```python
from build123d import *

# Parameters (mm, degrees)
BASE_FLANGE1_DEPTH          = 3.2639
F_1_4_START                 = -3.2639
F_1_4_CLEARANCE_SLOT1_DEPTH = 3.2639
SKETCH9_W                   = 1.5875
SKETCH9_H                   = 50.8
CUT_EXTRUDE1_DEPTH          = 274.80079868
FILLET1_R                   = 6.35
FILLET2_R                   = 19.05
FILLET3_R                   = 6.35
FILLET4_R                   = 1.5875
F_1_4_CLEARANCE_SLOT2_DEPTH = 3.2639
F_1_4_CLEARANCE_SLOT3_DEPTH = 3.2639


# Read off the part's stored shape, not the designer's step: 1/4 Clearance Slot1, 1/4 Clearance Slot2, 1/4 Clearance Slot3
# Sheet-metal steps are written as plain solids
with BuildPart() as part:
    # Sketch1 → Base-Flange1 (new body)
    with BuildSketch(Plane(origin=(0, 0, 0), x_dir=(0, 0, -1), z_dir=(1, 0, 0))):
        Polygon((38.1, 0), (38.1, -50.8), (201.36805286, 143.775288552), (151.652495469, 185.491594423), (38.1, 50.165), (38.1, 120.015), (-38.1, 120.015), (-38.1, 50.165), (-151.652495469, 185.491594423), (-201.36805286, 143.775288552), (-38.1, -50.8), (-38.1, 0), align=None)
    extrude(amount=-BASE_FLANGE1_DEPTH)

    # 1/4 Clearance Slot1 outline → 1/4 Clearance Slot1 (cut)
    with BuildSketch(Plane.YZ.offset(F_1_4_START)):
        with BuildLine():
            Line((57.3532, -24.0157), (88.6968, -24.0157))
            ThreePointArc((88.6968, -24.0157), (92.075, -20.6375), (88.6968, -17.2593))
            Line((88.6968, -17.2593), (57.3532, -17.2593))
            ThreePointArc((57.3532, -17.2593), (53.975, -20.6375), (57.3532, -24.0157))
        make_face()
        with BuildLine():
            Line((57.3532, 17.2593), (88.6968, 17.2593))
            ThreePointArc((88.6968, 17.2593), (92.075, 20.6375), (88.6968, 24.0157))
            Line((88.6968, 24.0157), (57.3532, 24.0157))
            ThreePointArc((57.3532, 24.0157), (53.975, 20.6375), (57.3532, 17.2593))
        make_face()
    extrude(amount=F_1_4_CLEARANCE_SLOT1_DEPTH, mode=Mode.SUBTRACT)

    # Sketch9 → Cut-Extrude1 (cut, through all)
    with BuildSketch(Plane(origin=(0, 0, 0), x_dir=(0, 0, -1), z_dir=(1, 0, 0))):
        with Locations((-38.89375, -25.4)):
            Rectangle(SKETCH9_W, SKETCH9_H)
        with Locations((38.89375, -25.4)):
            Rectangle(SKETCH9_W, SKETCH9_H)
    extrude(amount=-CUT_EXTRUDE1_DEPTH, mode=Mode.SUBTRACT)

    # Fillet1
    fillet1_edges = [part.edges().sort_by_distance(p)[0] for p in [
        (-1.63195, 185.491594423, -151.652495469),
        (-1.63195, 143.775288552, -201.36805286),
        (-1.63195, 143.775288552, 201.36805286),
        (-1.63195, 185.491594423, 151.652495469),
        (-1.63195, -48.908091172, 39.6875),
        (-1.63195, -48.908091172, -39.6875),
    ]]
    fillet(fillet1_edges, radius=FILLET1_R)

    # Fillet2
    fillet2_edges = [part.edges().sort_by_distance(p)[0] for p in [
        (-1.63195, 50.165, -38.1),
        (-1.63195, 50.165, 38.1),
    ]]
    fillet(fillet2_edges, radius=FILLET2_R)

    # Fillet3
    fillet3_edges = [part.edges().sort_by_distance(p)[0] for p in [
        (-1.63195, 120.015, 38.1),
        (-1.63195, 120.015, -38.1),
    ]]
    fillet(fillet3_edges, radius=FILLET3_R)

    # Fillet4
    fillet4_edges = [part.edges().sort_by_distance(p)[0] for p in [
        (-1.63195, 0, 39.6875),
        (-1.63195, 0, -39.6875),
    ]]
    fillet(fillet4_edges, radius=FILLET4_R)

    # 1/4 Clearance Slot2 outline → 1/4 Clearance Slot2 (cut)
    with BuildSketch(Plane.YZ.offset(F_1_4_START)):
        with BuildLine():
            Line((105.870311236, -102.982051315), (81.859720628, -82.834773592))
            ThreePointArc((81.859720628, -82.834773592), (77.100404187, -83.251159826), (77.516790422, -88.010476267))
            Line((77.516790422, -88.010476267), (101.527381029, -108.15775399))
            ThreePointArc((101.527381029, -108.15775399), (106.28669747, -107.741367756), (105.870311236, -102.982051315))
        make_face()
        with BuildLine():
            ThreePointArc((140.232307194, -131.81518945), (135.472990753, -132.231575685), (135.889376988, -136.990892126))
            Line((135.889376988, -136.990892126), (159.899967595, -157.138169849))
            ThreePointArc((159.899967595, -157.138169849), (164.659284036, -156.721783614), (164.242897801, -151.962467173))
            Line((164.242897801, -151.962467173), (140.232307194, -131.81518945))
        make_face()
        with BuildLine():
            Line((85.461804628, -127.303962384), (61.451214021, -107.156684661))
            ThreePointArc((61.451214021, -107.156684661), (56.69189758, -107.573070895), (57.108283815, -112.332387336))
            Line((57.108283815, -112.332387336), (81.118874422, -132.479665059))
            ThreePointArc((81.118874422, -132.479665059), (85.878190863, -132.063278825), (85.461804628, -127.303962384))
        make_face()
        with BuildLine():
            ThreePointArc((119.823800586, -156.137100519), (115.064484146, -156.553486754), (115.48087038, -161.312803195))
            Line((115.48087038, -161.312803195), (139.491460988, -181.460080918))
            ThreePointArc((139.491460988, -181.460080918), (144.250777428, -181.043694683), (143.834391194, -176.284378242))
            Line((143.834391194, -176.284378242), (119.823800586, -156.137100519))
        make_face()
    extrude(amount=F_1_4_CLEARANCE_SLOT2_DEPTH, mode=Mode.SUBTRACT)

    # 1/4 Clearance Slot3 outline → 1/4 Clearance Slot3 (cut)
    with BuildSketch(Plane.YZ.offset(F_1_4_START)):
        with BuildLine():
            Line((61.451214021, 107.156684661), (85.461804628, 127.303962384))
            ThreePointArc((85.461804628, 127.303962384), (85.878190863, 132.063278825), (81.118874422, 132.479665059))
            Line((81.118874422, 132.479665059), (57.108283815, 112.332387336))
            ThreePointArc((57.108283815, 112.332387336), (56.69189758, 107.573070895), (61.451214021, 107.156684661))
        make_face()
        with BuildLine():
            ThreePointArc((143.834391194, 176.284378242), (144.250777428, 181.043694683), (139.491460988, 181.460080918))
            Line((139.491460988, 181.460080918), (115.48087038, 161.312803195))
            ThreePointArc((115.48087038, 161.312803195), (115.064484146, 156.553486754), (119.823800586, 156.137100519))
            Line((119.823800586, 156.137100519), (143.834391194, 176.284378242))
        make_face()
        with BuildLine():
            Line((81.859720628, 82.834773592), (105.870311236, 102.982051315))
            ThreePointArc((105.870311236, 102.982051315), (106.28669747, 107.741367756), (101.527381029, 108.15775399))
            Line((101.527381029, 108.15775399), (77.516790422, 88.010476267))
            ThreePointArc((77.516790422, 88.010476267), (77.100404187, 83.251159826), (81.859720628, 82.834773592))
        make_face()
        with BuildLine():
            ThreePointArc((164.242897801, 151.962467173), (164.659284036, 156.721783614), (159.899967595, 157.138169849))
            Line((159.899967595, 157.138169849), (135.889376988, 136.990892126))
            ThreePointArc((135.889376988, 136.990892126), (135.472990753, 132.231575685), (140.232307194, 131.81518945))
            Line((140.232307194, 131.81518945), (164.242897801, 151.962467173))
        make_face()
    extrude(amount=F_1_4_CLEARANCE_SLOT3_DEPTH, mode=Mode.SUBTRACT)


solid = part.part
```
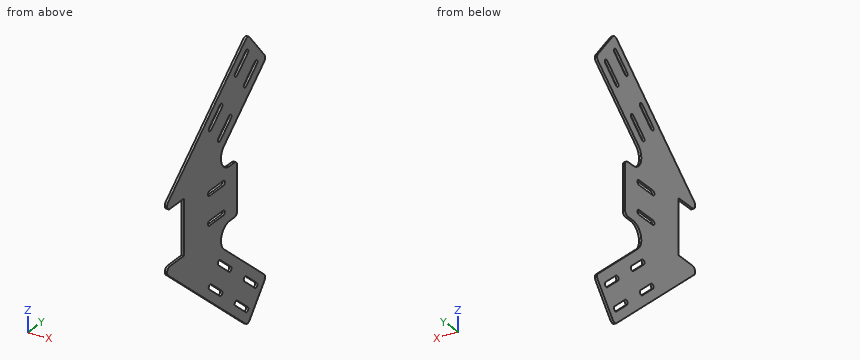
Part model, mm, in its own coordinate system. Round coordinates to 2 decimals unless told otherwise and drop trailing zeros. Write each loop counter-clockwise with the first axis right and the second up, starting at its lowest first coordinate (ties: lowest second). Pieces come first, ordered by that corner, then holes. Notation, with made-up numbers: (6.5, 37.5) -> (65.5, 37.5) arc R10 ccw to (65.5, 44.5) -> close; hole circle Ø11 at (46, 66.25). An arc over 180 degrees is marked (long way). Return JSON: item names as keys, results as strings. Group by question number.
Q1. Saw through at C-C on y = 153.5. Write the cut outline in (x, z).
Q2. Pin check, flat tips, straight feed: pin 1 (1.6 mm diameter, centred on x = -1, y = 72, fed in from -Z); pin 2 (1.5 mm diameter, centred on x = -2.5, z = 93, fed in from -Y); pin 3 (1.6 mm diameter, centred on x = -1, y = -13, fed in from -Z). Stop position of each tip, or through.
Q3. Probe L1, parallel to Z at x = -1, y = 126; L2, parallel to Z at x = -1.7, y = 156; L3, parallel to Y at x = -2.5, z = -107. List the from-to ranges inside material, lowest first. Write a range as [from, to].
Q4. Saw through at B-B on z = -116.5. Write the cut outline in (x, y), plus the area to 3 significant figures.
Q5. Saw through at D-D on x = -0.5. State how many separate pieces and enclosed holes the cut face has, plus the area to 3 significant figures.
Q6. Saw through at A-A on y = -19. Write the cut outline in (x, z).
Answer:
{
 "1": {"outline": "(-3.26, -189.78) -> (0, -189.78) -> (0, -151.77) -> (-3.26, -151.77) -> close; (-3.26, -142.95) -> (0, -142.95) -> (0, -124.81) -> (-3.26, -124.81) -> close; (-3.26, 124.81) -> (0, 124.81) -> (0, 142.95) -> (-3.26, 142.95) -> close; (-3.26, 151.77) -> (0, 151.77) -> (0, 189.78) -> (-3.26, 189.78) -> close"},
 "2": {"pin 1": "z = -141.81", "pin 2": "y = 13.73", "pin 3": "z = -70.49"},
 "3": {"L1": "[-186.45, -170.14], [-161.32, -101.73], [101.73, 161.32], [170.14, 186.45]", "L2": "[-186.8, -153.87], [-145.05, -126.91], [126.91, 145.05], [153.87, 186.8]", "L3": "[31.31, 57.31], [61.25, 100.15], [106.76, 132.28]"},
 "4": {"outline": "(-3.26, 42.63) -> (0, 42.63) -> (0, 62.08) -> (-3.26, 62.08) -> close; (-3.26, 72.59) -> (0, 72.59) -> (0, 143.6) -> (-3.26, 143.6) -> close", "area": "295 mm2"},
 "5": {"separate pieces": "1", "enclosed holes": "10", "area": "35,400 mm2"},
 "6": {"outline": "(-3.26, -64.78) -> (0, -64.78) -> (0, -39.69) -> (-3.26, -39.69) -> close; (-3.26, 39.69) -> (0, 39.69) -> (0, 64.78) -> (-3.26, 64.78) -> close"}
}
